```python
from build123d import *

# Parameters (mm, degrees)
SKETCH_1_W             = 150
SKETCH_1_H             = 45.5
EXTRUDE_1_DEPTH        = 2
CUT_EXTRUDE_1_REACH    = 80.4
SKETCH_2_R             = 1.65
CHAMFER_1_SIZE         = 8
CUT_EXTRUDE_1139_REACH = 80.4
SKETCH_3_R             = 2.5
CUT_EXTRUDE_2_REACH    = 80.4
SKETCH_4_R             = 1.65
FILLET_1_R             = 5
SKETCH_5_W             = 62
SKETCH_5_H             = 38
EXTRUDE_2_DEPTH        = 2
EXTRUDE_3_DEPTH        = 2


with BuildPart() as part:
    # Sketch 1 → Extrude 1 (new body)
    with BuildSketch(Plane(origin=(0, 0, 0), x_dir=(1, 0, 0), z_dir=(0, 1, 0))):
        Rectangle(SKETCH_1_W, SKETCH_1_H)
    extrude(amount=EXTRUDE_1_DEPTH)

    # Sketch 2 → Cut-Extrude 1 (cut, up to next)
    with BuildSketch(Plane(origin=(0, 2, 0), x_dir=(1, 0, 0), z_dir=(0, 1, 0)), mode=Mode.PRIVATE) as cut_extrude_1_sk1:
        with Locations(Location((-60, 15, 0), (0, 0, 270))):
            Circle(SKETCH_2_R)
    cut_extrude_1_tool1 = extrude(cut_extrude_1_sk1.sketch, amount=-CUT_EXTRUDE_1_REACH, mode=Mode.PRIVATE) & part.part
    # Sketch 2 → Cut-Extrude 1 (cut, up to next)
    with BuildSketch(Plane(origin=(0, 2, 0), x_dir=(1, 0, 0), z_dir=(0, 1, 0)), mode=Mode.PRIVATE) as cut_extrude_1_sk2:
        with Locations(Location((-66, 7, 0), (0, 0, 270))):
            Circle(SKETCH_2_R)
    cut_extrude_1_tool2 = extrude(cut_extrude_1_sk2.sketch, amount=-CUT_EXTRUDE_1_REACH, mode=Mode.PRIVATE) & part.part
    # Sketch 2 → Cut-Extrude 1 (cut, up to next)
    with BuildSketch(Plane(origin=(0, 2, 0), x_dir=(1, 0, 0), z_dir=(0, 1, 0)), mode=Mode.PRIVATE) as cut_extrude_1_sk3:
        with Locations(Location((-54, 7, 0), (0, 0, 270))):
            Circle(SKETCH_2_R)
    cut_extrude_1_tool3 = extrude(cut_extrude_1_sk3.sketch, amount=-CUT_EXTRUDE_1_REACH, mode=Mode.PRIVATE) & part.part
    # Sketch 2 → Cut-Extrude 1 (cut, up to next)
    with BuildSketch(Plane(origin=(0, 2, 0), x_dir=(1, 0, 0), z_dir=(0, 1, 0)), mode=Mode.PRIVATE) as cut_extrude_1_sk4:
        with Locations(Location((-71, -7, 0), (0, 0, 270))):
            Circle(SKETCH_2_R)
    cut_extrude_1_tool4 = extrude(cut_extrude_1_sk4.sketch, amount=-CUT_EXTRUDE_1_REACH, mode=Mode.PRIVATE) & part.part
    # Sketch 2 → Cut-Extrude 1 (cut, up to next)
    with BuildSketch(Plane(origin=(0, 2, 0), x_dir=(1, 0, 0), z_dir=(0, 1, 0)), mode=Mode.PRIVATE) as cut_extrude_1_sk5:
        with Locations(Location((-59, -7, 0), (0, 0, 270))):
            Circle(SKETCH_2_R)
    cut_extrude_1_tool5 = extrude(cut_extrude_1_sk5.sketch, amount=-CUT_EXTRUDE_1_REACH, mode=Mode.PRIVATE) & part.part
    # Sketch 2 → Cut-Extrude 1 (cut, up to next)
    with BuildSketch(Plane(origin=(0, 2, 0), x_dir=(1, 0, 0), z_dir=(0, 1, 0)), mode=Mode.PRIVATE) as cut_extrude_1_sk6:
        with Locations(Location((-65, -15, 0), (0, 0, 270))):
            Circle(SKETCH_2_R)
    cut_extrude_1_tool6 = extrude(cut_extrude_1_sk6.sketch, amount=-CUT_EXTRUDE_1_REACH, mode=Mode.PRIVATE) & part.part
    cut_extrude_1_1 = cut_extrude_1_tool1.solids().sort_by_distance((-60, 2, -15))[0]
    add(cut_extrude_1_1, mode=Mode.SUBTRACT)
    cut_extrude_1_2 = cut_extrude_1_tool2.solids().sort_by_distance((-66, 2, -7))[0]
    add(cut_extrude_1_2, mode=Mode.SUBTRACT)
    cut_extrude_1_3 = cut_extrude_1_tool3.solids().sort_by_distance((-54, 2, -7))[0]
    add(cut_extrude_1_3, mode=Mode.SUBTRACT)
    cut_extrude_1_4 = cut_extrude_1_tool4.solids().sort_by_distance((-71, 2, 7))[0]
    add(cut_extrude_1_4, mode=Mode.SUBTRACT)
    cut_extrude_1_5 = cut_extrude_1_tool5.solids().sort_by_distance((-59, 2, 7))[0]
    add(cut_extrude_1_5, mode=Mode.SUBTRACT)
    cut_extrude_1_6 = cut_extrude_1_tool6.solids().sort_by_distance((-65, 2, 15))[0]
    add(cut_extrude_1_6, mode=Mode.SUBTRACT)
    cut_extrude_1 = cut_extrude_1_1 + cut_extrude_1_2 + cut_extrude_1_3 + cut_extrude_1_4 + cut_extrude_1_5 + cut_extrude_1_6  # Cut-Extrude 1 as one shape, for the pattern or mirror that repeats it

    # Mirror 1: Cut-Extrude 1 across plane
    add(cut_extrude_1.mirror(Plane(origin=(0, 0, 0), x_dir=(0, 0, 1), z_dir=(1, 0, 0))), mode=Mode.SUBTRACT)

    # Chamfer 1
    chamfer_1_edges = [part.edges().sort_by_distance(p)[0] for p in [
        (75, 1, 22.75),
        (-75, 1, 22.75),
    ]]
    chamfer(chamfer_1_edges, length=CHAMFER_1_SIZE)

    # Sketch 3 → Cut-Extrude 1139 (cut, up to next)
    with BuildSketch(Plane(origin=(0, 2, 0), x_dir=(1, 0, 0), z_dir=(0, 1, 0)), mode=Mode.PRIVATE) as cut_extrude_1139_sk1:
        with Locations(Location((0, 0, 0), (0, 0, 270))):
            Circle(SKETCH_3_R)
    cut_extrude_1139_tool1 = extrude(cut_extrude_1139_sk1.sketch, amount=-CUT_EXTRUDE_1139_REACH, mode=Mode.PRIVATE) & part.part
    add(cut_extrude_1139_tool1.solids().sort_by_distance((0, 2, 0))[0], mode=Mode.SUBTRACT)

    # Sketch 4 → Cut-Extrude 2 (cut, up to next)
    with BuildSketch(Plane(origin=(0, 2, 0), x_dir=(1, 0, 0), z_dir=(0, 1, 0)), mode=Mode.PRIVATE) as cut_extrude_2_sk1:
        with Locations(Location((-40, 18, 0), (0, 0, 270))):
            Circle(SKETCH_4_R)
    cut_extrude_2_tool1 = extrude(cut_extrude_2_sk1.sketch, amount=-CUT_EXTRUDE_2_REACH, mode=Mode.PRIVATE) & part.part
    # Sketch 4 → Cut-Extrude 2 (cut, up to next)
    with BuildSketch(Plane(origin=(0, 2, 0), x_dir=(1, 0, 0), z_dir=(0, 1, 0)), mode=Mode.PRIVATE) as cut_extrude_2_sk2:
        with Locations(Location((-40, -18, 0), (0, 0, 270))):
            Circle(SKETCH_4_R)
    cut_extrude_2_tool2 = extrude(cut_extrude_2_sk2.sketch, amount=-CUT_EXTRUDE_2_REACH, mode=Mode.PRIVATE) & part.part
    # Sketch 4 → Cut-Extrude 2 (cut, up to next)
    with BuildSketch(Plane(origin=(0, 2, 0), x_dir=(1, 0, 0), z_dir=(0, 1, 0)), mode=Mode.PRIVATE) as cut_extrude_2_sk3:
        with Locations(Location((40, 18, 0), (0, 0, 270))):
            Circle(SKETCH_4_R)
    cut_extrude_2_tool3 = extrude(cut_extrude_2_sk3.sketch, amount=-CUT_EXTRUDE_2_REACH, mode=Mode.PRIVATE) & part.part
    # Sketch 4 → Cut-Extrude 2 (cut, up to next)
    with BuildSketch(Plane(origin=(0, 2, 0), x_dir=(1, 0, 0), z_dir=(0, 1, 0)), mode=Mode.PRIVATE) as cut_extrude_2_sk4:
        with Locations(Location((40, -18, 0), (0, 0, 270))):
            Circle(SKETCH_4_R)
    cut_extrude_2_tool4 = extrude(cut_extrude_2_sk4.sketch, amount=-CUT_EXTRUDE_2_REACH, mode=Mode.PRIVATE) & part.part
    add(cut_extrude_2_tool1.solids().sort_by_distance((-40, 2, -18))[0], mode=Mode.SUBTRACT)
    add(cut_extrude_2_tool2.solids().sort_by_distance((-40, 2, 18))[0], mode=Mode.SUBTRACT)
    add(cut_extrude_2_tool3.solids().sort_by_distance((40, 2, -18))[0], mode=Mode.SUBTRACT)
    add(cut_extrude_2_tool4.solids().sort_by_distance((40, 2, 18))[0], mode=Mode.SUBTRACT)

    # Fillet 1
    fillet_1_edges = [part.edges().sort_by_distance(p)[0] for p in [
        (75, 1, 14.75),
        (-75, 1, 14.75),
    ]]
    fillet(fillet_1_edges, radius=FILLET_1_R)

    # Sketch 5 → Extrude 2 (add)
    with BuildSketch(Plane(origin=(0, 0, 0), x_dir=(1, 0, 0), z_dir=(0, 1, 0))):
        with Locations((0, -41.75)):
            Rectangle(SKETCH_5_W, SKETCH_5_H)
    extrude(amount=EXTRUDE_2_DEPTH)

    # Sketch 6 → Extrude 3 (add)
    with BuildSketch(Plane(origin=(0, 0, 0), x_dir=(1, 0, 0), z_dir=(0, 1, 0))):
        Polygon((-31, -22.75), (-31, -34.75), (-39, -22.75), align=None)
        Polygon((31, -22.75), (31, -34.75), (39, -22.75), align=None)
    extrude(amount=EXTRUDE_3_DEPTH)


solid = part.part
```
Could you check a few things on this model? Use its own coordinates, in mm. Give positions to 0.01 mm unless a question says otherwise; leave off trailing zeros. Loops run counter-clockwise (first coordinate to the right, second up) from the corner with the lowest first, then second, coordinate; pieces in that order, holes last. Notation, with made-up numbers: (-13.5, -17.5) - (9.5, -17.5) arc R22 ccw to (9.5, 16.5) - close; hole circle Ø7 at (-4.5, 48). An arc over 180 degrees is marked (long way). Answer in a Markdown table with one row per item. Add a question column.
Q1. If we section it at B-B (x = -54): List the corners of the cut face in (y, z) for me.
Q2. If we section it at D-D (z = 54.5): List the corners of the cut face in (x, y) for me, plus the area to 3 significant figures.
Q3. We'd pull the mould along Z, two halves only. Please class faces 1 (the face through (60.6, 1, 6.6)), 2 (the face through (1, 0, 9)), 3 (the face through (34.944, 0.986, 28.834)): +Z half, -Z half, draft (parallel to the pull), parting line (faces both ways), or undercut.
Q4. Please list where these lines run through material, in increasing order: L1, parallel to X at y = 1.35, z = -15; L2, parallel to X at y = 1.2, z = 7; L3, parallel to X at y = 0.5, z = 18. Write a range as from..to.
Q5. If we section it at A-A (z = 0): List the corners of the cut face in (x, y) for me, plus the area to 3 significant figures.
Q6. If we section it at C-C (y = 1.3): State how many separate pieces and enclosed holes the cut face has, plus the area to 3 significant figures.
The answers:
| question | item | result |
|---|---|---|
| 1 | outline | (0, -22.75) - (2, -22.75) - (2, -8.65) - (0, -8.65) - close; (0, -5.35) - (2, -5.35) - (2, 22.75) - (0, 22.75) - close |
| 2 | outline | (-31, 0) - (31, 0) - (31, 2) - (-31, 2) - close |
| 2 | area | 124 mm^2 |
| 3 | face 1 | undercut |
| 3 | face 2 | draft |
| 3 | face 3 | +Z half |
| 4 | L1 | x = -75..-61.65, -58.35..58.35, 61.65..75 |
| 4 | L2 | x = -75..-72.65, -69.35..-60.65, -57.35..57.35, 60.65..69.35, 72.65..75 |
| 4 | L3 | x = -71.75..-41.65, -38.35..38.35, 41.65..71.75 |
| 5 | outline | (-75, 0) - (-2.5, 0) - (-2.5, 2) - (-75, 2) - close; (2.5, 0) - (75, 0) - (75, 2) - (2.5, 2) - close |
| 5 | area | 290 mm^2 |
| 6 | separate pieces | 1 |
| 6 | enclosed holes | 17 |
| 6 | area | 9,060 mm^2 |
